Could you check a few things on this model? Use its own coordinates, in mm. A direction names the side the tool comes from. Give positions to 0.01 mm unless a question says otherwise; leave off trailing zeros. Loops run counter-clockwise (first coordinate to the right, second up) from the corner with the lowest first, then second, coordinate; pieces in that order, holes last. Notation, with made-up numbers: (77.5, 16) - (127.5, 16) arc R35 cw to (127.5, 50) - close; hole circle Ø3 at (55, 1.5). An arc over 180 degrees is marked (long way). One line per item, written item: value. Start each with the question number.
Q1. I want a section at D-D (y = 45). Please give me the cut outline in (x, z), then the cut area to 4 significant figures.
Q2. I want a section at B-B (x = -60). Please give me the cut outline in (y, z).
Q3. I want a section at A-A (x = 32). Please give me the cut outline in (y, z), then the cut area to 3 significant figures.
Q4. If I drill on line 1 (Y direction, x = 29.5, z = -39); line 2 (X direction, y = -5, z = -8); line 3 (Y direction, x = -39, z = -28.5), over which ranges is the centre line in solid material (lowest first)? Write a range as from..to.
Q5. If we mould it in two halves opening along X, with no side actions, what happens to faces 6 (the face through (32, 12.5, -22)), 7 (the face through (-32.5, 9, -22)), 8 (the face through (52.99, 8.22, -22.82))? For each: released by +X, released by -X, zero draft, split by the parting line, or undercut.
Q6. I want a section at C-C (z = -5.5). Please give me the cut outline in (x, y), then the cut area to 3 significant figures.
Q7. For faces 1 (the face through (-60, 16.5, -22)), 2 (the face through (40, -37.5, -22)), 3 (the face through (12.28, 63.909, -17.505)), 4 (the face through (-22.5, 50, -22)), 5 (the face through (8.67, 74.444, -13.263)), which set-ups out of +Z, -Z, +X, -X, +Y, -Y let a thin tool reach every point of the face, with its end or its side?
Q8. I'm going to push flat-ended pins straight in: P1, Ø8, axis at x = -47.5, z = -25, coming from the +Y side; P2, Ø4, axis at y = -22.5, z = -17, coming from the +X side; P3, Ø1.5, axis at x = -41.5, z = -6.5, coming from the -Y side; P4, Ø2, axis at x = -23, z = -12, coming from the -Y side. Where does each tip first touch, or does it pass through?
```python
from build123d import *

# Parameters (mm, degrees)
SKETCH1_W           = 45
SKETCH1_H           = 115
BOSS_EXTRUDE1_DEPTH = 45
SKETCH2_W           = 45
SKETCH2_H           = 20
BOSS_EXTRUDE2_DEPTH = 35
BOSS_EXTRUDE3_DEPTH = 45
SKETCH4_R           = 10
BOSS_EXTRUDE4_DEPTH = 11
SKETCH4_3_R         = 5
BOSS_EXTRUDE5_DEPTH = 13
SKETCH6_R           = 10
BOSS_EXTRUDE6_DEPTH = 11
SKETCH7_R           = 10
BOSS_EXTRUDE7_DEPTH = 11
FILLET1_R           = 20
FILLET2_R           = 8
FILLET3_R           = 15
FILLET4_R           = 3


with BuildPart() as part:
    # Sketch1 → Boss-Extrude1 (new body)
    with BuildSketch(Plane.XY):
        Rectangle(SKETCH1_W, SKETCH1_H)
    extrude(amount=-BOSS_EXTRUDE1_DEPTH)

    # Sketch2 → Boss-Extrude2 (add)
    with BuildSketch(Plane(origin=(22.5, 0, 0), x_dir=(0, 0, -1), z_dir=(1, 0, 0))):
        with Locations((22.5, -47.5)):
            Rectangle(SKETCH2_W, SKETCH2_H)
        with Locations((22.5, 2.5)):
            Rectangle(SKETCH2_W, SKETCH2_H)
    extrude(amount=BOSS_EXTRUDE2_DEPTH)

    # Sketch3 → Boss-Extrude3 (add)
    with BuildSketch(Plane.XY):
        Polygon((-22.5, -17.5), (-32.5, -17.5), (-32.5, 27.5), (-87.5, 27.5), (-87.5, 42.5), (-22.5, 42.5), align=None)
    extrude(amount=-BOSS_EXTRUDE3_DEPTH)

    # Sketch4 → Boss-Extrude4 (add)
    with BuildSketch(Plane(origin=(0, 57.5, 0), x_dir=(1, 0, 0), z_dir=(0, 1, 0))):
        with Locations(Location((-8.5, 22.5, 0), (0, 0, 270))):
            Circle(SKETCH4_R)
    extrude(amount=BOSS_EXTRUDE4_DEPTH)

    # Sketch4<3> → Boss-Extrude5 (add)
    with BuildSketch(Plane(origin=(0, 57.5, 0), x_dir=(1, 0, 0), z_dir=(0, 1, 0))):
        with Locations(Location((12.5, 22.5, 0), (0, 0, 90))):
            Circle(SKETCH4_3_R)
    extrude(amount=BOSS_EXTRUDE5_DEPTH)

    # Sketch6 → Boss-Extrude6 (add)
    with BuildSketch(Plane(origin=(0, 70.5, 0), x_dir=(1, 0, 0), z_dir=(0, 1, 0))):
        with Locations(Location((12.5, 22.5, 0), (0, 0, 270))):
            Circle(SKETCH6_R)
    extrude(amount=BOSS_EXTRUDE6_DEPTH)

    # Sketch7 → Boss-Extrude7 (add)
    with BuildSketch(Plane.XZ.offset(-27.5)):
        with Locations((-60, -22.5)):
            Circle(SKETCH7_R)
    extrude(amount=BOSS_EXTRUDE7_DEPTH)

    # Fillet1
    fillet1_edges = [part.edges().sort_by_distance(p)[0] for p in [
        (-87.5, 35, 0),
        (-87.5, 35, -45),
    ]]
    fillet(fillet1_edges, radius=FILLET1_R)

    # Fillet2
    fillet2_edges = [part.edges().sort_by_distance(p)[0] for p in [
        (-32.5, -17.5, -22.5),
    ]]
    fillet(fillet2_edges, radius=FILLET2_R)

    # Fillet3
    fillet3_edges = [part.edges().sort_by_distance(p)[0] for p in [
        (57.5, -57.5, -22.5),
        (57.5, 12.5, -22.5),
    ]]
    fillet(fillet3_edges, radius=FILLET3_R)

    # Fillet4
    fillet4_edges = [part.edges().sort_by_distance(p)[0] for p in [
        (-8.5, 68.5, -32.5),
        (12.5, 81.5, -32.5),
        (-70, 16.5, -22.5),
    ]]
    fillet(fillet4_edges, radius=FILLET4_R)


solid = part.part
```
Worked answers:
1. outline: (-22.5, -45) - (22.5, -45) - (22.5, 0) - (-22.5, 0) - close
1. area: 2,025 mm²
2. outline: (16.5, -29.5) arc R3 ccw to (19.5, -32.5) - (27.5, -32.5) - (27.5, -45) - (42.5, -45) - (42.5, 0) - (27.5, 0) - (27.5, -12.5) - (19.5, -12.5) arc R3 ccw to (16.5, -15.5) - close
3. outline: (-57.5, -45) - (-37.5, -45) - (-37.5, 0) - (-57.5, 0) - close; (-7.5, -45) - (12.5, -45) - (12.5, 0) - (-7.5, 0) - close
3. area: 1,800 mm²
4. line 1: y = -57.5..-37.5, -7.5..12.5
4. line 2: x = -32.5..57.5
4. line 3: y = 27.5..42.5
5. face 6: zero draft
5. face 7: undercut
5. face 8: released by +X
6. outline: (-81.27, 27.5) - (-32.5, 27.5) - (-32.5, -9.5) arc R8 ccw to (-24.5, -17.5) - (-22.5, -17.5) - (-22.5, -57.5) - (42.5, -57.5) arc R15 ccw to (57.5, -42.5) - (57.5, -37.5) - (22.5, -37.5) - (22.5, -7.5) - (57.5, -7.5) - (57.5, -2.5) arc R15 ccw to (42.5, 12.5) - (22.5, 12.5) - (22.5, 57.5) - (-22.5, 57.5) - (-22.5, 42.5) - (-81.27, 42.5) - close
6. area: 7,800 mm²
7. face 1: +Z, -Z, -X, -Y
7. face 2: +Z, -Z, +X
7. face 3: none
7. face 4: +Z, -Z, -X, +Y
7. face 5: +Y
8. P1: stops at y = 42.5
8. P2: stops at x = 22.5
8. P3: stops at y = 27.5
8. P4: stops at y = -57.5
